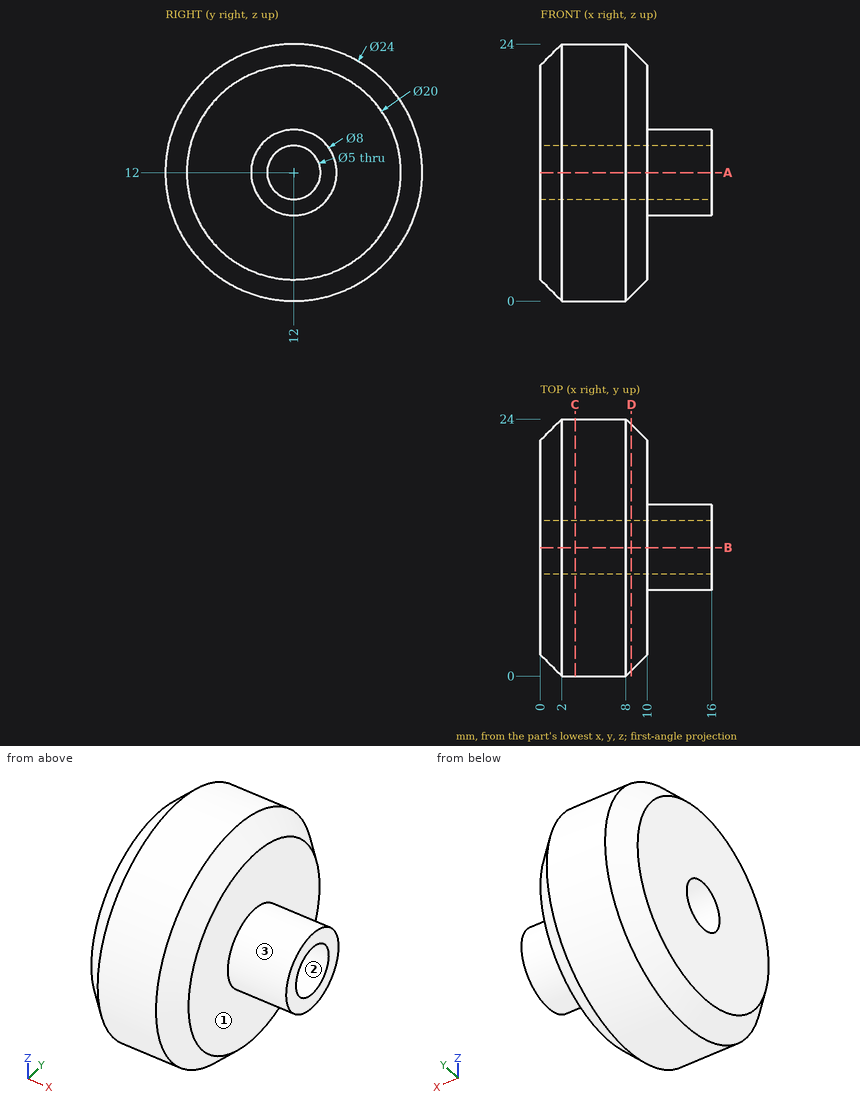
Could you check a few things on this drawing? It's one solid part, dimensions in mm from its lowest x, y, z. Coordinates: 2 decimals unless noted, no trailing zeros. Loops run counter-clockwise (first coordinate to the right, second up) from the corner with the lowest first, then second, coordinate; pieces in that order, holes last.
1. We'd pull the mould along Y, two halves only. Please class the marked faces 1, 2 and 3: released by +Y, released by -Y, zero draft, split by the parting line, or undercut.
2. I need wall thicknesses on L1, parallel to X at y = 18.25, z = 6.25; L2, parallel to Z at x = 8.25, y = 13.5; L3, parallel to Y at x = 12, z = 12. Which ranges of each line are inside material? Lowest first, please.
3. Imagine slicing it at C-C (x = 3.25). Please give me the cut outline in (y, z).
4. Imagine slicing it at D-D (x = 8.5). Please give me the cut outline in (y, z), and give its area (3 significant figures).
5. For P1, Ø4, axis at y = 4, z = 5.5, coming from the +X side; P2, Ø6, axis at x = 10.5, y = 7, coming from the -Z side; P3, Ø2, axis at x = 10, y = 8, coming from the +Z side; P4, Ø2, axis at y = 18, z = 20.5, coming from the -X side, each with a flat end and sliding along its axis, tell me the tip position at first contact or that it passes through.
6. Imagine slicing it at A-A (z = 12). Please give me the cut outline in (x, y).
Computed values:
1. face 1: zero draft
1. face 2: undercut
1. face 3: split by the parting line
2. L1: x = 0 to 10
2. L2: z = 0.35 to 10, 14 to 23.65
2. L3: y = 8 to 9.5, 14.5 to 16
3. outline: circle Ø24 at (12, 12); hole circle Ø5 at (12, 12)
4. outline: circle Ø23 at (12, 12); hole circle Ø5 at (12, 12)
4. area: 396 mm2
5. P1: stops at x = 10
5. P2: stops at z = 0.47
5. P3: stops at z = 22.31
5. P4: stops at x = 0
6. outline: (0, 2) - (2, 0) - (8, 0) - (10, 2) - (10, 8) - (16, 8) - (16, 9.5) - (0, 9.5) - close; (0, 14.5) - (16, 14.5) - (16, 16) - (10, 16) - (10, 22) - (8, 24) - (2, 24) - (0, 22) - close
